```python
from build123d import *

# Parameters (mm, degrees)
SKETCH_1_W               = 100
SKETCH_1_H               = 180
EXTRUDE_1_DEPTH          = 100
SKETCH_2_W               = 50
SKETCH_2_H               = 68.6
CUT_EXTRUDE_1_DEPTH      = 90
SKETCH_3_W               = 170
SKETCH_3_H               = 90
CUT_EXTRUDE_2_DEPTH      = 101
SKETCH_4_R               = 3.25
CUT_EXTRUDE_3_DEPTH      = 1
CUT_EXTRUDE_3_DEPTH_BACK = 181


with BuildPart() as part:
    # 草图1 → 凸台-拉伸1 (new body)
    with BuildSketch(Plane(origin=(0, 0, 0), x_dir=(1, 0, 0), z_dir=(0, 1, 0))):
        Rectangle(SKETCH_1_W, SKETCH_1_H)
    extrude(amount=EXTRUDE_1_DEPTH)

    # 草图2 → 切除-拉伸1 (cut)
    with BuildSketch(Plane(origin=(0, 100, 0), x_dir=(1, 0, 0), z_dir=(0, 1, 0))):
        with Locations((-15, 44.3)):
            Rectangle(SKETCH_2_W, SKETCH_2_H)
    extrude(amount=-CUT_EXTRUDE_1_DEPTH, mode=Mode.SUBTRACT)

    # 草图3 → 切除-拉伸2 (cut, through all)
    with BuildSketch(Plane.ZY.offset(50)):
        with Locations((0, 50)):
            Rectangle(SKETCH_3_W, SKETCH_3_H)
    extrude(amount=-CUT_EXTRUDE_2_DEPTH, mode=Mode.SUBTRACT)

    # 草图4 → 切除-拉伸3 (cut, two sides)
    with BuildSketch(Plane.XY.offset(90)) as cut_extrude_3_sk:
        with Locations((-15, 50)):
            Circle(SKETCH_4_R)
    extrude(amount=CUT_EXTRUDE_3_DEPTH, mode=Mode.SUBTRACT)
    extrude(cut_extrude_3_sk.sketch, amount=-CUT_EXTRUDE_3_DEPTH_BACK, mode=Mode.SUBTRACT)


solid = part.part
```
The listing builds one solid part. Answer for the finished solid, in the listing's coordinates (mm). A direction names the side the tool comes from. Coordinates: 2 decimals unless noted, no trailing zeros. Loops run counter-clockwise (first coordinate to the right, second up) from the corner with the lowest first, then second, coordinate; pieces in that order, holes last. Notation, with made-up numbers: (0.25, 63.25) - (12.25, 63.25) arc R17 cw to (12.25, 80.25) - close; hole circle Ø10 at (-23.75, -3). An arc over 180 degrees is marked (long way). Use a Markdown table: item, result. Add a question column.
1) The part is cut by section D-D, the plane y = 62.5. Give the vertices of the cut face in (x, z).
2) The part is cut by section A-A, the plane y = 50. Give the vertices of the cut face in (x, z).
3) The mould has two halves that part along X. Classify faces 4 (the flat face through (50, 98, 7)), 5 (the cylindrical face through (-15.705, 46.827, -87.465)), 6 (the flat face through (-1, 5, -1)): released by +X, released by -X, zero draft, split by the parting line, or undercut.
4) The part is cut by section B-B, the plane x = -15. Give the vertices of the cut face in (y, z).
5) For faces 1 (the flat face through (-1, 49, -90)), 2 (the flat face through (-1, 49, 85)), 3 (the flat face through (10, 98, -44)), determine the directions among +Z, -Z, +X, -X, +Y, -Y from which every point of the face is accessible in a straight line to the end or side of a thin tool.
6) The part is cut by section C-C, the plane z = -17. Give the vertices of the cut face in (x, y).
7) Find the intervals of material crossed by line 1 (Y direction, x = -15, z = -88); line 2 (Y direction, x = -17, z = 8); line 3 (Z direction, x = -31, y = 68), in increasing order.
Here are the results:
| question | item | result |
|---|---|---|
| 1 | outline | (-50, -90) - (50, -90) - (50, -85) - (-50, -85) - close; (-50, 85) - (50, 85) - (50, 90) - (-50, 90) - close |
| 2 | outline | (-50, -90) - (-18.25, -90) - (-18.25, -85) - (-50, -85) - close; (-50, 85) - (-18.25, 85) - (-18.25, 90) - (-50, 90) - close; (-11.75, -90) - (50, -90) - (50, -85) - (-11.75, -85) - close; (-11.75, 85) - (50, 85) - (50, 90) - (-11.75, 90) - close |
| 3 | face 4 | released by +X |
| 3 | face 5 | undercut |
| 3 | face 6 | zero draft |
| 4 | outline | (0, -90) - (46.75, -90) - (46.75, -85) - (5, -85) - (5, 85) - (46.75, 85) - (46.75, 90) - (0, 90) - close; (53.25, -90) - (100, -90) - (100, -78.6) - (95, -78.6) - (95, -85) - (53.25, -85) - close; (53.25, 85) - (95, 85) - (95, -10) - (100, -10) - (100, 90) - (53.25, 90) - close |
| 5 | face 1 | -Z, +X, -X, +Y, -Y |
| 5 | face 2 | +X, -X |
| 5 | face 3 | +Y |
| 6 | outline | (-50, 0) - (50, 0) - (50, 5) - (-50, 5) - close; (-50, 95) - (-40, 95) - (-40, 100) - (-50, 100) - close; (10, 95) - (50, 95) - (50, 100) - (10, 100) - close |
| 7 | line 1 | y = 0 to 46.75, 53.25 to 100 |
| 7 | line 2 | y = 0 to 5, 95 to 100 |
| 7 | line 3 | z = -90 to -85, 85 to 90 |
